from build123d import *

# Parameters (mm, degrees)
CUT_EXTRUDE1_DEPTH = 2


with BuildPart() as part:
    # Sketch1 → Revolve1 (revolve)
    with BuildSketch(Plane.XY, mode=Mode.PRIVATE) as revolve1_sk:
        with BuildLine():
            Line((0, 0), (0, 2.625))
            ThreePointArc((0, 2.625), (0.256281566, 3.243718434), (0.875, 3.5))
            Line((0.875, 3.5), (4, 3.5))
            Line((4, 3.5), (4, 2))
            Line((4, 2), (39, 2))
            Line((39, 2), (39, 0))
            Line((39, 0), (0, 0))
        make_face()
    revolve(revolve1_sk.sketch.rotate(Axis((0, 0, 0), (1, 0, 0)), 180), axis=Axis((0, 0, 0), (1, 0, 0)))

    # Sketch2 → Cut-Extrude1 (cut)
    with BuildSketch(Plane.ZY):
        Polygon((0, 1.732050808), (-1.5, 0.866025404), (-1.5, -0.866025404), (0, -1.732050808), (1.5, -0.866025404), (1.5, 0.866025404), align=None)
    extrude(amount=-CUT_EXTRUDE1_DEPTH, mode=Mode.SUBTRACT)


solid = part.part
Check sheet for the modelled part. Datum: model origin and axes. Units: mm. A direction names the side the tool comes from. Coordinates: 2 decimals unless noted, no trailing zeros. Write each loop counter-clockwise with the first axis right and the second up, starting at its lowest first coordinate (ties: lowest second). Pieces come first, ordered by that corner, then holes.
Item 1: Cross-section at B-B on x = 26. Record the boundary of the cut face in (y, z).
Numbers:
outline: circle Ø4 at (0, 0)
Item 2: Cross-section at A-A on y = 0. Record the boundary of the cut face in (x, z) (3 decimals).
Numbers:
outline: (0, -2.625) arc R0.875 ccw to (0.875, -3.5) - (4, -3.5) - (4, -2) - (39, -2) - (39, 2) - (4, 2) - (4, 3.5) - (0.875, 3.5) arc R0.875 ccw to (0, 2.625) - (0, 1.5) - (2, 1.5) - (2, -1.5) - (0, -1.5) - close
Item 3: Depth check by flat-ended pin: pin 1 Ø3 at (x, z) = (18, 2.5) entering from -Y; pin 2 Ø1.4 at (x, y) = (1, -0.5) entering from +Z; pin 3 Ø1 at (x, y) = (18, -0.5) entering from +Z; pin 4 Ø2 at (x, z) = (5.5, -2.5) entering from -Y. Enter the tip coordinate at first touch or a pass-through.
Numbers:
pin 1: stops at y = -1.73
pin 2: stops at z = 3.5
pin 3: stops at z = 2
pin 4: stops at y = -1.32
Item 4: Scan lines: probe 1 along Y at (x, z) = (7, -1); probe 2 along X at (y, z) = (-1.5, 2.25). Record each from-to range of solid material in increasing order.
Numbers:
probe 1: y = -1.73 to 1.73
probe 2: x = 0 to 4
Item 5: Access from +Z, -Z, +X, -X, +Y, -Y to the whole of each face (thin tool, end or side, straight path). Record for faces 1 (the face through (39, 0, 0)), 2 (the face through (4, -2, 2)), 3 (the face through (0.986, 1.305, -0.74)).
Numbers:
face 1: +Z, -Z, +X, +Y, -Y
face 2: +X
face 3: -X
Item 6: Mould release check, pull along Z, two halves, no side actions. Record for faces 4 (the face through (0.986, -1.293, -0.76)), 5 (the face through (0, 0, 2)), 6 (the face through (22, 0, 2)): released by +Z, released by -Z, zero draft, split by the parting line, or undercut.
Numbers:
face 4: undercut
face 5: zero draft
face 6: split by the parting line
